Input: part model. Units: mm. Frame: model coordinates. Face numbers are marked on the shaded views. A direction names the side the tool comes from. Give positions to 0.01 mm unless a question says otherwise; leave off trailing zeros. Loops run counter-clockwise (first coordinate to the right, second up) from the corner with the lowest first, then second, coordinate; pieces in that order, holes last.
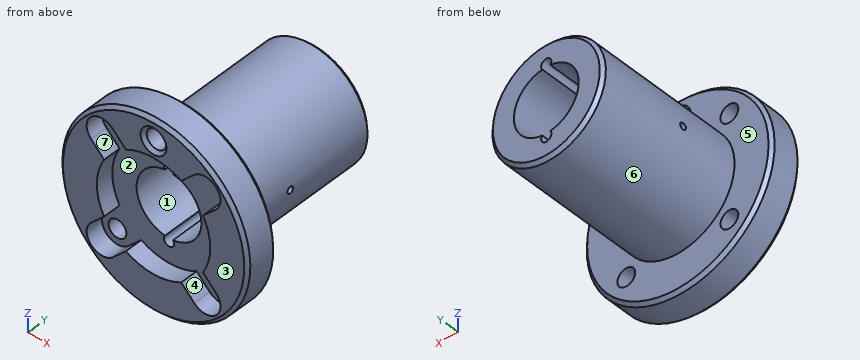
from build123d import *
from build123d.topology import SkipClean

# Parameters (mm, degrees)
SKETCH_1_R               = 29
EXTRUDE_1_DEPTH          = 10
SKETCH_2_R               = 17.5
EXTRUDE_2_DEPTH          = 56
SKETCH_3_R               = 10
CUT_EXTRUDE_1_DEPTH      = 56
CUT_EXTRUDE_2_REACH      = 71.412
SKETCH_4_R               = 2.75
SKETCH_4_R_2             = 3
SKETCH_4_4_R             = 4.75
SKETCH_4_4_R_2           = 2.75
CUT_EXTRUDE_3_DEPTH      = 5.4
SKETCH_3_3_R             = 10
SKETCH_3_3_R_2           = 1.585
CUT_EXTRUDE_4_DEPTH      = 56
CUT_EXTRUDE_5_DEPTH      = 70.411814556
CUT_EXTRUDE_5_DEPTH_BACK = 70.411814556
SKETCH_9_R               = 1
CUT_EXTRUDE_6_DEPTH      = 5.4
CHAMFER_1_SIZE           = 1
CHAMFER_2_SIZE           = 1
CHAMFER_3_SIZE           = 1


with BuildPart() as part:
    # 草图1 → 凸台-拉伸1 (new body)
    with BuildSketch(Plane(origin=(0, 0, 0), x_dir=(1, 0, 0), z_dir=(0, 1, 0))):
        with Locations(Location((0, 0, 0), (0, 0, 270))):
            Circle(SKETCH_1_R)
    extrude(amount=EXTRUDE_1_DEPTH)

    # 草图2 → 凸台-拉伸2 (add)
    with BuildSketch(Plane(origin=(0, 0, 0), x_dir=(1, 0, 0), z_dir=(0, 1, 0))):
        with Locations(Location((0, 0, 0), (0, 0, 270))):
            Circle(SKETCH_2_R)
    extrude(amount=EXTRUDE_2_DEPTH)

    # 草图3 → 切除-拉伸1 (cut)
    with BuildSketch(Plane(origin=(0, 0, 0), x_dir=(1, 0, 0), z_dir=(0, 1, 0))):
        with Locations(Location((0, 0, 0), (0, 0, 270))):
            Circle(SKETCH_3_R)
    extrude(amount=CUT_EXTRUDE_1_DEPTH, mode=Mode.SUBTRACT)

    # 草图4 → 切除-拉伸2 (cut, up to next)
    with BuildSketch(Plane.XZ, mode=Mode.PRIVATE) as cut_extrude_2_sk1:
        with Locations(Location((-15.909902577, 15.909902577, 0), (0, 0, 270))):
            Circle(SKETCH_4_R)
    cut_extrude_2_tool1 = extrude(cut_extrude_2_sk1.sketch, amount=-CUT_EXTRUDE_2_REACH, mode=Mode.PRIVATE) & part.part
    # 草图4 → 切除-拉伸2 (cut, up to next)
    with BuildSketch(Plane.XZ, mode=Mode.PRIVATE) as cut_extrude_2_sk2:
        with Locations(Location((-15.909902577, -15.909902577, 0), (0, 0, 270))):
            Circle(SKETCH_4_R)
    cut_extrude_2_tool2 = extrude(cut_extrude_2_sk2.sketch, amount=-CUT_EXTRUDE_2_REACH, mode=Mode.PRIVATE) & part.part
    # 草图4 → 切除-拉伸2 (cut, up to next)
    with BuildSketch(Plane.XZ, mode=Mode.PRIVATE) as cut_extrude_2_sk3:
        with Locations(Location((15.909902577, -15.909902577, 0), (0, 0, 270))):
            Circle(SKETCH_4_R)
    cut_extrude_2_tool3 = extrude(cut_extrude_2_sk3.sketch, amount=-CUT_EXTRUDE_2_REACH, mode=Mode.PRIVATE) & part.part
    # 草图4 → 切除-拉伸2 (cut, up to next)
    with BuildSketch(Plane.XZ, mode=Mode.PRIVATE) as cut_extrude_2_sk4:
        with Locations(Location((15.909902577, 15.909902577, 0), (0, 0, 270))):
            Circle(SKETCH_4_R)
    cut_extrude_2_tool4 = extrude(cut_extrude_2_sk4.sketch, amount=-CUT_EXTRUDE_2_REACH, mode=Mode.PRIVATE) & part.part
    # 草图4 → 切除-拉伸2 (cut, up to next)
    with BuildSketch(Plane.XZ, mode=Mode.PRIVATE) as cut_extrude_2_sk5:
        with Locations(Location((0, 22.5, 0), (0, 0, 270))):
            Circle(SKETCH_4_R_2)
    cut_extrude_2_tool5 = extrude(cut_extrude_2_sk5.sketch, amount=-CUT_EXTRUDE_2_REACH, mode=Mode.PRIVATE) & part.part
    add(cut_extrude_2_tool1.solids().sort_by_distance((-15.909903, 0, 15.909903))[0], mode=Mode.SUBTRACT)
    add(cut_extrude_2_tool2.solids().sort_by_distance((-15.909903, 0, -15.909903))[0], mode=Mode.SUBTRACT)
    add(cut_extrude_2_tool3.solids().sort_by_distance((15.909903, 0, -15.909903))[0], mode=Mode.SUBTRACT)
    add(cut_extrude_2_tool4.solids().sort_by_distance((15.909903, 0, 15.909903))[0], mode=Mode.SUBTRACT)
    add(cut_extrude_2_tool5.solids().sort_by_distance((0, 0, 22.5))[0], mode=Mode.SUBTRACT)

    # 草图4<4> → 切除-拉伸3 (cut)
    # profile 1 of 4: a face of its own
    with BuildSketch(Plane.XZ):
        with Locations(Location((-15.909902577, 15.909902577, 0), (0, 0, 270))):
            Circle(SKETCH_4_4_R)
        with Locations(Location((-15.909902577, 15.909902577, 0), (0, 0, 270))):
            Circle(SKETCH_4_4_R_2, mode=Mode.SUBTRACT)
    # profile 2 of 4: a face of its own
    with BuildSketch(Plane.XZ):
        with Locations(Location((15.909902577, 15.909902577, 0), (0, 0, 270))):
            Circle(SKETCH_4_4_R)
        with Locations(Location((15.909902577, 15.909902577, 0), (0, 0, 270))):
            Circle(SKETCH_4_4_R_2, mode=Mode.SUBTRACT)
    # profile 3 of 4: a face of its own
    with BuildSketch(Plane.XZ):
        with Locations(Location((15.909902577, -15.909902577, 0), (0, 0, 270))):
            Circle(SKETCH_4_4_R)
        with Locations(Location((15.909902577, -15.909902577, 0), (0, 0, 270))):
            Circle(SKETCH_4_4_R_2, mode=Mode.SUBTRACT)
    # profile 4 of 4: a face of its own
    with BuildSketch(Plane.XZ):
        with Locations(Location((-15.909902577, -15.909902577, 0), (0, 0, 270))):
            Circle(SKETCH_4_4_R)
        with Locations(Location((-15.909902577, -15.909902577, 0), (0, 0, 270))):
            Circle(SKETCH_4_4_R_2, mode=Mode.SUBTRACT)
    extrude(amount=-CUT_EXTRUDE_3_DEPTH, mode=Mode.SUBTRACT)

    # 草图3<3> → 切除-拉伸4 (cut)
    with BuildSketch(Plane(origin=(0, 0, 0), x_dir=(1, 0, 0), z_dir=(0, 1, 0))):
        Circle(SKETCH_3_3_R)
        with Locations((0, -10.9)):
            Circle(SKETCH_3_3_R_2)
        with Locations((0, 10.9)):
            Circle(SKETCH_3_3_R_2)
    extrude(amount=CUT_EXTRUDE_4_DEPTH, mode=Mode.SUBTRACT)

    # 草图9 → 切除-拉伸5 (cut, two sides: drawn at the far end of the back side and taken through both)
    with SkipClean():  # the faces are left unmerged after this step: merging them gives an invalid solid
        with BuildSketch(Plane(origin=(0, 0, 0), x_dir=(0, 0, -1), z_dir=(1, 0, 0)).offset(-CUT_EXTRUDE_5_DEPTH_BACK)):
            with Locations((0, 28)):
                Circle(SKETCH_9_R)
        extrude(amount=CUT_EXTRUDE_5_DEPTH + CUT_EXTRUDE_5_DEPTH_BACK, mode=Mode.SUBTRACT)

    # 草图11 → 切除-拉伸6 (cut)
    with BuildSketch(Plane(origin=(0, 0, 0), x_dir=(1, 0, 0), z_dir=(0, 1, 0))):
        with BuildLine():
            Line((-19.268659787, 12.551145366), (-15.26857459, 8.551060168))
            ThreePointArc((-15.26857459, 8.551060168), (-17.5, 0), (-15.26857459, -8.551060168))
            Line((-15.26857459, -8.551060168), (-19.268659787, -12.551145366))
            Line((-19.268659787, -12.551145366), (-12.551145366, -19.268659787))
            Line((-12.551145366, -19.268659787), (-8.551060168, -15.26857459))
            ThreePointArc((-8.551060168, -15.26857459), (0, -17.5), (8.551060168, -15.26857459))
            Line((8.551060168, -15.26857459), (12.551145366, -19.268659787))
            Line((12.551145366, -19.268659787), (19.268659787, -12.551145366))
            Line((19.268659787, -12.551145366), (15.26857459, -8.551060168))
            ThreePointArc((15.26857459, -8.551060168), (17.5, 0), (15.26857459, 8.551060168))
            Line((15.26857459, 8.551060168), (19.268659787, 12.551145366))
            Line((19.268659787, 12.551145366), (12.551145366, 19.268659787))
            Line((12.551145366, 19.268659787), (8.551060168, 15.26857459))
            ThreePointArc((8.551060168, 15.26857459), (0, 17.5), (-8.551060168, 15.26857459))
            Line((-8.551060168, 15.26857459), (-12.551145366, 19.268659787))
            Line((-12.551145366, 19.268659787), (-19.268659787, 12.551145366))
        make_face()
    extrude(amount=CUT_EXTRUDE_6_DEPTH, mode=Mode.SUBTRACT)

    # 倒角1
    chamfer_1_edges = [part.edges().sort_by_distance(p)[0] for p in [
        (0, 0, -29),
        (0, 10, -29),
        (0, 56, -17.5),
    ]]
    chamfer(chamfer_1_edges, length=CHAMFER_1_SIZE)

    # 倒角2
    chamfer_2_edges = [part.edges().sort_by_distance(p)[0] for p in [
        (0, 0, 25.5),
    ]]
    chamfer(chamfer_2_edges, length=CHAMFER_2_SIZE)

    # 倒角3
    chamfer_3_edges = [part.edges().sort_by_distance(p)[0] for p in [
        (0, 10, 25.5),
    ]]
    chamfer(chamfer_3_edges, length=CHAMFER_3_SIZE)


solid = part.part
(1) Mould query, pull axis Z, two halves, no side actions, for the marked faces 4, 5, 6 and 7. Classes: +Z half, -Z half, draft (parallel to the pull), parting line (faces both ways), or undercut.
Values follow:
face 4: undercut
face 5: draft
face 6: parting line
face 7: undercut
(2) Reachability of the marked faces 1, 2 and 3 from +Z, -Z, +X, -X, +Y, -Y: full face, straight path, thin tool, end or side. Return the list, or none.
Values follow:
face 1: +Y, -Y
face 2: -Y
face 3: +Z, -Z, +X, -X, -Y
(3) Cut plane A-A (x = 0). Count the separate pieces of the cut face and the enclosed holes in it, and give its area (3 significant figures).
Values follow:
separate pieces: 3
enclosed holes: 0
area: 673 mm2
(4) Cut plane C-C (y = 20.5). Return the cut outline in (x, z) (3 decimals).
Values follow:
outline: circle Ø35 at (0, 0); hole (-1.247, -9.922) arc R1.585 ccw (long way) to (1.247, -9.922) arc R10 ccw to (1.247, 9.922) arc R1.585 ccw (long way) to (-1.247, 9.922) arc R10 ccw to start
(5) Ray query, probe 1 along Z at (x, y) = (0, 18) (3 decimals); probe 2 along Y at (x, z) = (12.5, 0); probe 3 along Y at (x, z) = (16.5, 13). Return the intervals inside material, ascending.
Values follow:
probe 1: z = -17.5 to -12.485, 12.485 to 17.5
probe 2: y = 5.4 to 27, 29 to 56
probe 3: y = 5.4 to 10
(6) Pin query (flat end, axial travel): pin 1 Ø2.5 at (y, z) = (28, 0) entering from -X; pin 2 Ø6.5 at (x, z) = (15.91, 15.91) entering from +Y; pin 3 Ø4 at (x, z) = (0, -10.9) entering from -Y; pin 4 Ø12 at (x, z) = (0.5, 12) entering from -Y. Return the tip coordinate at first contact, or that it passes through.
Values follow:
pin 1: stops at x = -17.5
pin 2: stops at y = 10
pin 3: stops at y = 5.4
pin 4: stops at y = 0
(7) Cut plane D-D (y = 28). Return the cut outline in (x, z) (3 decimals), and give its area (3 significant figures).
Values follow:
outline: (-17.471, -1) arc R17.5 ccw to (17.471, -1) - (9.95, -1) arc R10 cw to (1.247, -9.922) arc R1.585 cw (long way) to (-1.247, -9.922) arc R10 cw to (-9.95, -1) - close; (-17.471, 1) - (-9.95, 1) arc R10 cw to (-1.247, 9.922) arc R1.585 cw (long way) to (1.247, 9.922) arc R10 cw to (9.95, 1) - (17.471, 1) arc R17.5 ccw to start
area: 605 mm2
